```python
from build123d import *

# Parameters (mm, degrees)
SKETCH_1_R          = 3
EXTRUDE_2_DEPTH     = 1
SKETCH_3_R          = 1.5
CUT_EXTRUDE_1_DEPTH = 10
SKETCH_5_R          = 1.5
CUT_EXTRUDE_2_DEPTH = 1


with BuildPart() as part:
    # 草图1 → 凸台-拉伸2 (new body)
    with BuildSketch(Plane.XY):
        Polygon((-10, 50.109212084), (10, 50.109212084), (60, -28.838156337), (60, -49.890787916), (-60, -49.890787916), (-60, -29.890787916), align=None)
        with Locations((-50, -39.890787916)):
            Circle(SKETCH_1_R, mode=Mode.SUBTRACT)
        with Locations((50, -39.890787916)):
            Circle(SKETCH_1_R, mode=Mode.SUBTRACT)
    extrude(amount=EXTRUDE_2_DEPTH)

    # 草图3 → 切除-拉伸1 (cut)
    with BuildSketch(Plane.XY.offset(1)):
        with Locations((-11.15, 31.109212084)):
            Circle(SKETCH_3_R)
        with Locations((11.15, 31.109212084)):
            Circle(SKETCH_3_R)
    extrude(amount=-CUT_EXTRUDE_1_DEPTH, mode=Mode.SUBTRACT)

    # 草图5 → 切除-拉伸2 (cut)
    with BuildSketch(Plane.XY.offset(1)):
        with Locations((25, -14.890787916)):
            Circle(SKETCH_5_R)
        with Locations((25, -44.890787916)):
            Circle(SKETCH_5_R)
        with Locations(Location((-25, -44.890787916, 0), (0, 0, 180))):
            Circle(SKETCH_5_R)
        with Locations(Location((-25, -14.890787916, 0), (0, 0, 180))):
            Circle(SKETCH_5_R)
    extrude(amount=-CUT_EXTRUDE_2_DEPTH, mode=Mode.SUBTRACT)


solid = part.part
```
The listing builds one solid part. Answer for the finished solid, in the listing's coordinates (mm). Coordinates: 2 decimals unless noted, no trailing zeros. Write each loop counter-clockwise with the first axis right and the second up, starting at its lowest first coordinate (ties: lowest second). Pieces come first, ordered by that corner, then holes. Notation, with made-up numbers: (11.5, -14) - (52.5, -14) arc R12 cw to (52.5, -7) - close; hole circle Ø4 at (-12, -26). An arc over 180 degrees is marked (long way). Return JSON: item names as keys, results as strings. Group by question number.
Q1. The part is cut by section A-A on x = -25. Write down the section's boundary in (y, z), and give its area (3 significant figures).
Q2. Flat-ended cylindrical pins translate along their axes: pin 1 Ø4 at (x, y) = (-11.15, 31.11) entering from -Z; pin 2 Ø2.5 at (x, y) = (-25, -44.89) entering from -Z. Find the tip coordinate at first contact, or state that the pin passes through.
Q3. Find the intervals of material crossed by line 1 along X through (y, z) = (-40, 0.35); line 2 along Y through (x, z) = (-25, 0.6); line 3 along X through (y, z) = (-44.5, 0.75), in increasing order. Write a range as [from, to].
Q4. The part is cut by section B-B on z = 0.15. State how many separate pieces and enclosed holes the cut face has, and give its area (3 significant figures).
Q5. For a pull along X with two mould halves and no side action, classify faces 1 (the cylindrical face through (-23.89, -15.9, 0.51)), 2 (the flat face through (-35.35, 9.55, 0.49)), 3 (the flat face through (1, -10, 0)), 4 (the cylindrical face through (-53, -39.8, 0.5)) as +X half, -X half, draft (parallel to the pull), parting line (faces both ways), or undercut.
Q6. The part is cut by section D-D on y = -19.5. Write down the section's boundary in (x, z), and give its area (3 significant figures).
Q7. The part is cut by section C-C on x = 50. Write down the section's boundary in (y, z).
Evaluation:
{
 "1": {"outline": "(-49.89, 0) - (-46.39, 0) - (-46.39, 1) - (-49.89, 1) - close; (-43.39, 0) - (-16.39, 0) - (-16.39, 1) - (-43.39, 1) - close; (-13.39, 0) - (26.11, 0) - (26.11, 1) - (-13.39, 1) - close", "area": "70.0 mm2"},
 "2": {"pin 1": "stops at z = 0", "pin 2": "passes through"},
 "3": {"line 1": "x = [-60, -53], [-47, 47], [53, 60]", "line 2": "y = [-49.89, -46.39], [-43.39, -16.39], [-13.39, 26.11]", "line 3": "x = [-60, -26.45], [-23.55, 23.55], [26.45, 60]"},
 "4": {"separate pieces": "1", "enclosed holes": "8", "area": "7,930 mm2"},
 "5": {"face 1": "undercut", "face 2": "-X half", "face 3": "draft", "face 4": "undercut"},
 "6": {"outline": "(-53.51, 0) - (54.09, 0) - (54.09, 1) - (-53.51, 1) - close", "area": "108 mm2"},
 "7": {"outline": "(-49.89, 0) - (-42.89, 0) - (-42.89, 1) - (-49.89, 1) - close; (-36.89, 0) - (-13.05, 0) - (-13.05, 1) - (-36.89, 1) - close"}
}
